Here's how the part is built. I have some questions about the finished solid (model axes, mm). A direction names the side the tool comes from. Coordinates: 2 decimals unless noted, no trailing zeros. Write each loop counter-clockwise with the first axis right and the second up, starting at its lowest first coordinate (ties: lowest second). Pieces come first, ordered by that corner, then holes. Notation, with made-up numbers: (87.5, 11) -> (117.5, 11) arc R11 ccw to (117.5, 17) -> close; hole circle Ø10 at (73.5, 6.25). An arc over 180 degrees is marked (long way). Put each result on its own line as item: value.
```python
from build123d import *

# Parameters (mm, degrees)
ESQUISSE2_W                           = 60
ESQUISSE2_H                           = 30
T_LE_DE_BASE_PLI_E1_DEPTH             = 1
T_LE_PLI_E_SUR_AR_TE1_STRIP_W         = 5.4732
T_LE_PLI_E_SUR_AR_TE1_STRIP_H         = 1
T_LE_PLI_E_SUR_AR_TE1_STRIP_CUT_DEPTH = 30
T_LE_PLI_E_SUR_AR_TE1_DEPTH           = 30
T_LE_PLI_E_SUR_AR_TE2_STRIP_W         = 5.4732
T_LE_PLI_E_SUR_AR_TE2_STRIP_H         = 1
T_LE_PLI_E_SUR_AR_TE2_STRIP_CUT_DEPTH = 30
T_LE_PLI_E_SUR_AR_TE2_DEPTH           = 30
ENL_V_MAT_EXTRU_1_DEPTH               = 44.462627624
ENL_V_MAT_EXTRU_2_REACH               = 45.463
ESQUISSE27_R                          = 1.7
ESQUISSE29_R                          = 1.7
ENL_V_MAT_EXTRU_3_DEPTH               = 44.289721644


# Sheet-metal steps are written as plain solids
with BuildPart() as part:
    # Esquisse2 → Tôle de base pliée1 (new body)
    with BuildSketch(Plane(origin=(0, 0, 0), x_dir=(1, 0, 0), z_dir=(0, 1, 0))):
        Rectangle(ESQUISSE2_W, ESQUISSE2_H)
    extrude(amount=-T_LE_DE_BASE_PLI_E1_DEPTH)

    # Tôle pliée sur arête1 strip (across the edge) → Tôle pliée sur arête1 strip cut (cut)
    with BuildSketch(Plane(origin=(30, -1, -15), x_dir=(-1, 0, 0), z_dir=(0, 0, 1))):
        with Locations((-2, -0.5)):
            Rectangle(T_LE_PLI_E_SUR_AR_TE1_STRIP_W, T_LE_PLI_E_SUR_AR_TE1_STRIP_H)
    extrude(amount=T_LE_PLI_E_SUR_AR_TE1_STRIP_CUT_DEPTH, mode=Mode.SUBTRACT)

    # Tôle pliée sur arête1 section (across the edge) → Tôle pliée sur arête1 (add)
    with BuildSketch(Plane(origin=(30, -1, -15), x_dir=(-1, 0, 0), z_dir=(0, 0, 1))):
        with BuildLine():
            Line((-1, 0.7366), (-1, 6))
            Line((-1, 6), (0, 6))
            Line((0, 6), (0, 0.7366))
            ThreePointArc((0, 0.7366), (0.215745145, 0.215745145), (0.7366, 0))
            Line((0.7366, 0), (0.7366, -1))
            ThreePointArc((0.7366, -1), (-0.491361636, -0.491361636), (-1, 0.7366))
        make_face()
    extrude(amount=T_LE_PLI_E_SUR_AR_TE1_DEPTH)

    # Tôle pliée sur arête2 strip (across the edge) → Tôle pliée sur arête2 strip cut (cut)
    with BuildSketch(Plane(origin=(30, -7, -15), x_dir=(0, 1, 0), z_dir=(0, 0, 1))):
        with Locations((-2, -0.5)):
            Rectangle(T_LE_PLI_E_SUR_AR_TE2_STRIP_W, T_LE_PLI_E_SUR_AR_TE2_STRIP_H)
    extrude(amount=T_LE_PLI_E_SUR_AR_TE2_STRIP_CUT_DEPTH, mode=Mode.SUBTRACT)

    # Tôle pliée sur arête2 section (across the edge) → Tôle pliée sur arête2 (add)
    with BuildSketch(Plane(origin=(30, -7, -15), x_dir=(0, 1, 0), z_dir=(0, 0, 1))):
        with BuildLine():
            Line((-1, 0.7366), (-1, 70))
            Line((-1, 70), (0, 70))
            Line((0, 70), (0, 0.7366))
            ThreePointArc((0, 0.7366), (0.215745145, 0.215745145), (0.7366, 0))
            Line((0.7366, 0), (0.7366, -1))
            ThreePointArc((0.7366, -1), (-0.491361636, -0.491361636), (-1, 0.7366))
        make_face()
    extrude(amount=T_LE_PLI_E_SUR_AR_TE2_DEPTH)

    # Esquisse26 → Enlèv. mat.-Extru.1 (cut, through all)
    with BuildSketch(Plane(origin=(0, 0, 0), x_dir=(1, 0, 0), z_dir=(0, 1, 0))):
        with BuildLine():
            Line((-17.5, 7.5), (7.5, 7.5))
            ThreePointArc((7.5, 7.5), (15, 0), (7.5, -7.5))
            Line((7.5, -7.5), (-17.5, -7.5))
            ThreePointArc((-17.5, -7.5), (-25, 0), (-17.5, 7.5))
        make_face()
    extrude(amount=-ENL_V_MAT_EXTRU_1_DEPTH, mode=Mode.SUBTRACT)

    # Esquisse27 → Enlèv. mat.-Extru.2 (cut, up to next)
    with BuildSketch(Plane(origin=(0, -8, 0), x_dir=(1, 0, 0), z_dir=(0, 1, 0)), mode=Mode.PRIVATE) as enl_v_mat_extru_2_sk1:
        with Locations(Location((-35, 10, 0), (0, 0, 180))):
            Circle(ESQUISSE27_R)
    enl_v_mat_extru_2_tool1 = extrude(enl_v_mat_extru_2_sk1.sketch, amount=ENL_V_MAT_EXTRU_2_REACH, mode=Mode.PRIVATE) & part.part
    # Esquisse27 → Enlèv. mat.-Extru.2 (cut, up to next)
    with BuildSketch(Plane(origin=(0, -8, 0), x_dir=(1, 0, 0), z_dir=(0, 1, 0)), mode=Mode.PRIVATE) as enl_v_mat_extru_2_sk2:
        with Locations((-35, -10)):
            Circle(ESQUISSE27_R)
    enl_v_mat_extru_2_tool2 = extrude(enl_v_mat_extru_2_sk2.sketch, amount=ENL_V_MAT_EXTRU_2_REACH, mode=Mode.PRIVATE) & part.part
    add(enl_v_mat_extru_2_tool1.solids().sort_by_distance((-35, -8, -10))[0], mode=Mode.SUBTRACT)
    add(enl_v_mat_extru_2_tool2.solids().sort_by_distance((-35, -8, 10))[0], mode=Mode.SUBTRACT)

    # Esquisse29 → Enlèv. mat.-Extru.3 (cut, through all)
    with BuildSketch(Plane(origin=(0, -7, 0), x_dir=(1, 0, 0), z_dir=(0, 1, 0))):
        with Locations(Location((26, 0, 0), (0, 0, 180))):
            Circle(ESQUISSE29_R)
    extrude(amount=-ENL_V_MAT_EXTRU_3_DEPTH, mode=Mode.SUBTRACT)


solid = part.part
```
Item 1: For P1, Ø3.5, axis at y = -3, z = -6, coming from the -X side; P2, Ø5.5, axis at x = -35, z = 10, coming from the +Y side; P3, Ø1, axis at y = -1, z = 0.5, coming from the +X side, each with a flat end and sliding along its axis, tell me the tip position at first contact or that it passes through.
Output:
P1: stops at x = 29.82
P2: stops at y = -7
P3: stops at x = 30.98
Item 2: Which directions (+Z, -Z, +X, -X, +Y, -Y) give clear straight access to the entire face, cutting with the end or side of a thin tool? Please do faces 4 (the flat face through (-6, -7, -10)), 5 (the cylindrical face through (24.43, -7.49, -0.65)), 6 (the cylindrical face through (15, -7.49, -0.16)).
Output:
face 4: +Z, -Z, -X
face 5: -Y
face 6: +Y, -Y
Item 3: Imagine slicing it at B-B on x = 26. Write out the boundary of the cut face in (y, z), then the cut area to 3 significant figures.
Output:
outline: (-8, -15) -> (-7, -15) -> (-7, -1.7) -> (-8, -1.7) -> close; (-8, 1.7) -> (-7, 1.7) -> (-7, 15) -> (-8, 15) -> close; (-1, -15) -> (0, -15) -> (0, 15) -> (-1, 15) -> close
area: 56.6 mm²
Item 4: Imagine slicing it at C-C on z = 0. Write out the boundary of the cut face in (x, y), then the cut area to 3 significant figures.
Output:
outline: (-40, -8) -> (-25, -8) -> (-25, -7) -> (-40, -7) -> close; (-30, -1) -> (-25, -1) -> (-25, 0) -> (-30, 0) -> close; (15, -8) -> (24.3, -8) -> (24.3, -7) -> (15, -7) -> close; (15, -1) -> (29.26, -1) arc R0.74 cw to (30, -1.74) -> (30, -6.26) arc R0.74 cw to (29.26, -7) -> (27.7, -7) -> (27.7, -8) -> (29.26, -8) arc R1.74 ccw to (31, -6.26) -> (31, -1.74) arc R1.74 ccw to (29.26, 0) -> (15, 0) -> close
area: 53.5 mm²
Item 5: Imagine slicing it at D-D on x = 4. Write out the boundary of the cut face in (y, z).
Output:
outline: (-8, -15) -> (-7, -15) -> (-7, -7.5) -> (-8, -7.5) -> close; (-8, 7.5) -> (-7, 7.5) -> (-7, 15) -> (-8, 15) -> close; (-1, -15) -> (0, -15) -> (0, -7.5) -> (-1, -7.5) -> close; (-1, 7.5) -> (0, 7.5) -> (0, 15) -> (-1, 15) -> close
Item 6: If we mould it in two halves opening along X, with no side actions, what happens to faces 1 (the cylindrical face through (-34.2, -7.5, 11.5)), 2 (the flat face through (31, -4, 0)), 3 (the flat face through (-2, -7.2, -15))? For each: released by +X, released by -X, zero draft, split by the parting line, or undercut.
Output:
face 1: undercut
face 2: released by +X
face 3: zero draft
Item 7: Imagine slicing it at A-A on z = -4.5. Write out the boundary of the cut face in (x, y), then the cut area to 3 significant figures.
Output:
outline: (-40, -8) -> (-23.5, -8) -> (-23.5, -7) -> (-40, -7) -> close; (-30, -1) -> (-23.5, -1) -> (-23.5, 0) -> (-30, 0) -> close; (13.5, -8) -> (29.26, -8) arc R1.74 ccw to (31, -6.26) -> (31, -1.74) arc R1.74 ccw to (29.26, 0) -> (13.5, 0) -> (13.5, -1) -> (29.26, -1) arc R0.74 cw to (30, -1.74) -> (30, -6.26) arc R0.74 cw to (29.26, -7) -> (13.5, -7) -> close
area: 62.9 mm²
Item 8: Please list where these lines run through material, in increasing order: line 1 along Z through (x, y) = (26, -7.4); line 2 along Z through (x, y) = (-35, -7.65); line 3 along Y through (x, z) = (-18.5, -10.5). Write a range as from..to.
Output:
line 1: z = -15..-1.7, 1.7..15
line 2: z = -15..-11.7, -8.3..8.3, 11.7..15
line 3: y = -8..-7, -1..0
